```python
from build123d import *

# Parameters (mm, degrees)
F0_R     = 15
F1_DEPTH = 30
F2_W     = 20
F2_H     = 20
F3_DEPTH = 25
F4_W     = 20
F4_H     = 20
F5_DEPTH = 7
F6_W     = 10
F6_H     = 11.633402
F7_DEPTH = 20


with BuildPart() as f1:
    # F0 (on Front) → F1 (new body)
    with BuildSketch(Plane.XZ):
        Circle(F0_R)
    extrude(amount=F1_DEPTH)

    # F2 (on face) → F3 (cut)
    with BuildSketch(Plane.XZ.offset(30)):
        Rectangle(F2_W, F2_H)
    extrude(amount=-F3_DEPTH, mode=Mode.SUBTRACT)

    # F4 (on Right) → F5 (join)
    with BuildSketch(Plane.YZ):
        with Locations((-17.3568, 21.899901)):
            Rectangle(F4_W, F4_H)
    extrude(amount=F5_DEPTH)

    # F6 (on face) → F7 (cut)
    with BuildSketch(Plane.YZ.offset(7)):
        with Locations((-17.3568, 21.0832)):
            Rectangle(F6_W, F6_H)
    extrude(amount=-F7_DEPTH, mode=Mode.SUBTRACT)


solid = f1.part
```
CAD build for the part. Positions are in the model's coordinates, mm. A direction names the side the tool comes from. Coordinates: 2 decimals unless noted, no trailing zeros. Write each loop counter-clockwise with the first axis right and the second up, starting at its lowest first coordinate (ties: lowest second). Pieces come first, ordered by that corner, then holes. Notation, with made-up numbers: (62.25, 67.5) -> (103.25, 67.5) arc R16 cw to (103.25, 87.5) -> close; hole circle Ø6 at (82.25, -16.5). An arc over 180 degrees is marked (long way). Use CSV: the item, a comma, the result in double quotes. Start each with the question number.
Item 1: Wall check: probe 1 along Y at (x, z) = (-1, 5.5); probe 2 along X at (y, z) = (-8.5, -6.5); probe 3 along Z at (x, y) = (1.5, -18). Give the ranges that are in metal, low to high.
Item 2: Two-plate mould, pull along Y, no slides. Class faces 1 (the flat face through (4, -17, 15.266)), 2 (the flat face through (3, -7.357, 22)), 3 (the flat face through (-11, -30, 1)), 4 (the flat face through (10, -18, 0)): +Y half, -Y half, draft (parallel to the pull), parting line (faces both ways), or undercut.
Item 3: Band-saw the part on B-B, the plane y = -11. Write the cut outline in (x, z), plus the area to 3 significant figures.
Item 4: Band-saw the part on D-D, the plane z = -9. Write the cut outline in (x, y), plus the area to 3 significant figures.
Item 5: Tool access for faces 5 (the flat face through (-10, -18, 0)), 6 (the flat face through (0, -17.5, 27.3)), 7 (the flat face through (7, -17, 29)), 8 (the flat face through (4, -12.357, 21)): list every direction of +Z, -Z, +X, -X, +Y, -Y with a clear straight run to the whole face (end or side of a thin tool).
Item 6: Drop flat-ended pins along their axis: P1, Ø2, axis at y = -25, z = 21, coming from the -X side; P2, Ø5.5, axis at y = -18.5, z = 26.5, coming from the +X side; P3, Ø8, axis at x = 3, z = 1.5, coming from the +Y side; P4, Ø3, axis at y = -4.5, z = -9.5, coming from the -X side. Give the stop position or say it passes through.
Item 7: Band-saw the part on C-C, the plane z = 20. Write the cut outline in (x, y), plus the area to 3 significant figures.
Item 8: Band-saw the part on A-A, the plane y = -18.75. Write the cut outline in (x, z), plus the area to 3 significant figures.
Response values:
1,probe 1,"y = -5 to 0"
1,probe 2,"x = -13.52 to -10, 10 to 13.52"
1,probe 3,"z = -14.92 to -10, 10 to 15.27, 26.9 to 31.9"
2,face 1,"undercut"
2,face 2,"+Y half"
2,face 3,"-Y half"
2,face 4,"draft"
3,outline,"(0, 15) arc R15 ccw (long way) to (7, 13.27) -> (7, 31.9) -> (0, 31.9) -> close; hole (-10, -10) -> (10, -10) -> (10, 10) -> (-10, 10) -> close"
3,area,"429 mm2"
4,outline,"(-12, -30) -> (-10, -30) -> (-10, -5) -> (10, -5) -> (10, -30) -> (12, -30) -> (12, 0) -> (-12, 0) -> close"
4,area,"220 mm2"
5,face 5,"-Y"
5,face 6,"+Z, -X, +Y, -Y"
5,face 7,"+Z, +X, +Y, -Y"
5,face 8,"+X, -X"
6,P1,"stops at x = 0"
6,P2,"stops at x = 7"
6,P3,"stops at y = 0"
6,P4,"stops at x = -12.69"
7,outline,"(0, -27.36) -> (7, -27.36) -> (7, -22.36) -> (0, -22.36) -> close; (0, -12.36) -> (7, -12.36) -> (7, -7.36) -> (0, -7.36) -> close"
7,area,"70.0 mm2"
8,outline,"(0, 15) arc R15 ccw (long way) to (7, 13.27) -> (7, 15.27) -> (0, 15.27) -> close; (0, 26.9) -> (7, 26.9) -> (7, 31.9) -> (0, 31.9) -> close; hole (-10, -10) -> (10, -10) -> (10, 10) -> (-10, 10) -> close"
8,area,"348 mm2"
